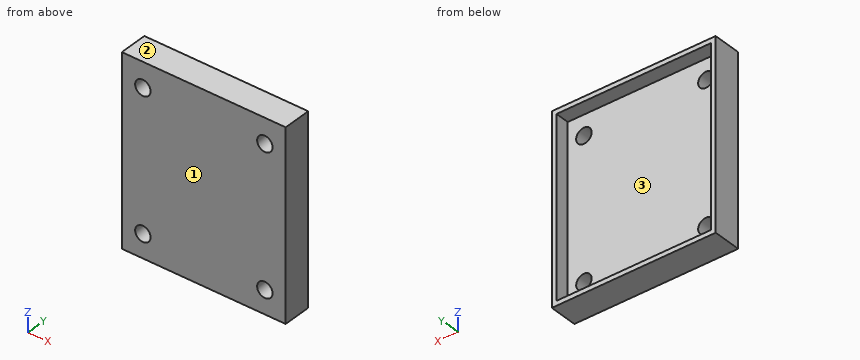
Autodesk Inventor part; units mm, degrees
ref_plane "YZ Plane" through (0, 0, 0) normal (1, 0, 0) x (0, 1, 0)
ref_plane "XZ Plane" through (0, 0, 0) normal (0, 1, 0) x (-1, 0, 0)
ref_plane "XY Plane" through (0, 0, 0) normal (0, 0, 1) x (1, 0, 0)
sketch "Sketch1" plane through (0, 0, 0) normal (0, 1, 0) x (-1, 0, 0)
  line L0 (4.6706, 7.7326) -> (-28.3294, 7.7326)
  line L1 (-28.3294, 7.7326) -> (-28.3294, -32.2674)
  line L2 (-28.3294, -32.2674) -> (4.6706, -32.2674)
  line L3 (4.6706, -32.2674) -> (4.6706, 7.7326)
  point P0 (0, 0)
  dimension "d0" = 33
  dimension "d1" = 40
extrude "Extrusion1" add sketch "Sketch1" along normal blind 3
sketch "Sketch2" plane through (0, 3, 0) normal (0, 1, 0) x (1, 0, 0)
  line L0 (-4.6706, 32.2674) -> (-4.6706, -7.7326)
  line L1 (-4.6706, -7.7326) -> (-4.6706, -4.7326)
  line L2 (-4.6706, -4.7326) -> (-2.8206, -4.7326)
  line L3 (-2.8206, -4.7326) -> (-2.8206, 28.2674)
  line L4 (-2.8206, 28.2674) -> (26.4794, 28.2674)
  line L5 (26.4794, 28.2674) -> (26.4794, -4.7326)
  line L6 (-2.8206, -4.7326) -> (-1.1706, -4.7326)
  line L7 (26.4794, -4.7326) -> (24.8794, -4.7326)
  line L8 (24.8794, -4.7326) -> (24.8794, 28.2674)
  line L9 (-2.8206, 28.2674) -> (-1.1706, 28.2674)
  line L10 (-1.1706, -4.7326) -> (-1.1706, -1.4326)
  line L11 (-1.1706, -1.4326) -> (24.8794, -1.4326)
  point P0 (0, 0)
  dimension "d4" = 3
  dimension "d5" = 1.85
  dimension "d6" = 90
  dimension "d7" = 33
  dimension "d8" = 29.3
  dimension "d9" = 1.65
  dimension "d10" = 1.6
  dimension "d11" = 1.65
  dimension "d26" = 3.3
hole "Hole1" at (-1.1706, 3, 1.4326) at (24.8794, 3, 1.4326) at (24.8794, 3, -28.2674) at (-1.1706, 3, -28.2674) direction (0, -1, 0) diameter 3.3 end through all
sketch "Sketch3" plane through (0, 0, 0) normal (0, -1, 0) x (1, 0, 0)
  line L0 (28.3294, -32.2674) -> (-4.6706, -32.2674)
  line L1 (-4.6706, -32.2674) -> (-5.6706, -32.2674)
  line L2 (-5.6706, -32.2674) -> (-5.6706, -33.2674)
  line L3 (-5.6706, -33.2674) -> (29.3294, -33.2674)
  line L4 (29.3294, -33.2674) -> (29.3294, 8.7326)
  line L5 (28.3294, 7.7326) -> (28.3294, -32.2674)
  line L6 (29.3294, 8.7326) -> (-5.6706, 8.7326)
  line L7 (-5.6706, 8.7326) -> (-5.6706, -32.2674)
  circle A0 centre (24.8794, -28.2674) radius 1.65
  circle A1 centre (-1.1706, -28.2674) radius 1.65
  line L8 (-4.6706, 7.7326) -> (28.3294, 7.7326)
  line L9 (-4.6706, -32.2674) -> (-4.6706, 7.7326)
  line L10 (28.3294, -32.2674) -> (-4.6706, -32.2674)
  line L11 (28.3294, 7.7326) -> (28.3294, -32.2674)
  point P0 (0, 0)
  dimension "d19" = 1
  dimension "d20" = 1
  dimension "d21" = 35
  dimension "d22" = 42
  dimension "d23" = 90
extrude "Extrusion2" add sketch "Sketch3" against normal blind 6 contours L7 L6 L4 L3 L2
sketch "Sketch4" plane through (-5.6706, 0, 8.7326) normal (0, 0, 1) x (1, 0, 0)
  point P0 (5.6706, 0)
sketch "Sketch5" plane through (0, 0, 0) normal (0, -1, 0) x (1, 0, 0)
  line L0 (-5.6706, -33.2674) -> (-5.6706, 8.7326)
  line L1 (-5.6706, 8.7326) -> (-5.6706, 5.7326)
  line L2 (-5.6706, 5.7326) -> (29.3294, 5.7326)
  line L3 (29.3294, -33.2674) -> (29.3294, 8.7326)
  line L4 (29.3294, 8.7326) -> (-5.6706, 8.7326)
  line L5 (-5.6706, 5.7326) -> (-5.6706, 6.7326)
  line L6 (-5.6706, 6.7326) -> (29.3294, 6.7326)
  line L7 (28.3294, 7.7326) -> (-4.6706, 7.7326)
  line L8 (29.3294, 6.7326) -> (29.3294, 5.7326)
  point P0 (0, 0)
  dimension "d27" = 3
  dimension "d28" = 1
extrude "Extrusion3" cut sketch "Sketch5" against normal blind 10 contours L0 L4 L3 L6
extrude "Extrusion4" add sketch "Sketch5" against normal blind 6 contours L0 L6 L3 L2
properties part number "testing holes for circuit board"
Verification items for the finished model (mm, model axes). Face numbers are marked on the shaded views. Coordinates: 2 decimals unless noted, no trailing zeros. Order: outer loops, then holes, each group sorted by start corner. A loop starts at its lowest first (then second) coordinate and runs counter-clockwise, first axis right, second up. Notation, with made-up numbers: (57, -29.5) -> (69, -29.5) arc R38 cw to (69, 8.5) -> close; hole circle Ø11 at (70, 55). An arc over 180 degrees is marked (long way). Use CSV: the item, a comma, the result in double quotes. Start each with the question number.
Q1. Depth check by flat-ended pin: P1, Ø1.5, axis at x = 8.5, z = -9, coming from the +Y side. Enter the tip coordinate at first touch or a pass-through.
Q2. Section check A-A, the plane y = 4.4. Record the cut outline in (x, z), and give its area (3 significant figures).
Q3. Section check C-C, the plane x = 0. Record the cut outline in (y, z), and give its area (3 significant figures).
Q4. Thickness scan on line 1 along X through (y, z) = (3.8, -22); line 2 along Z through (x, y) = (25, 4.45); line 3 along Z through (x, y) = (-2, 0.95). Record the ranges inside material, lowest first.
Q5. Draft check along Z on the marked faces 1, 2 and 3. Enter one of: +Z half, -Z half, draft (parallel to the pull), parting line (faces both ways), or undercut.
Q6. Section check D-D, the plane x = 12. Record the cut outline in (y, z), and give its area (3 significant figures).
Q7. Section check B-B, the plane z = -20. Record the cut outline in (x, y), and give its area (3 significant figures).
Returned:
1,P1,"stops at y = 3"
2,outline,"(-5.67, -33.27) -> (29.33, -33.27) -> (29.33, 6.73) -> (-5.67, 6.73) -> close; hole (-4.67, -32.27) -> (28.33, -32.27) -> (28.33, 5.73) -> (-4.67, 5.73) -> close"
2,area,"146 mm^2"
3,outline,"(0, -33.27) -> (6, -33.27) -> (6, -32.27) -> (3, -32.27) -> (3, -29.43) -> (0, -29.43) -> close; (0, -27.1) -> (3, -27.1) -> (3, 0.27) -> (0, 0.27) -> close; (0, 2.6) -> (3, 2.6) -> (3, 5.73) -> (6, 5.73) -> (6, 6.73) -> (0, 6.73) -> close"
3,area,"112 mm^2"
4,line 1,"x = -5.67 to -4.67, 28.33 to 29.33"
4,line 2,"z = -33.27 to -32.27, 5.73 to 6.73"
4,line 3,"z = -33.27 to -29.69, -26.84 to 0.01, 2.86 to 6.73"
5,face 1,"draft"
5,face 2,"+Z half"
5,face 3,"undercut"
6,outline,"(0, -33.27) -> (6, -33.27) -> (6, -32.27) -> (3, -32.27) -> (3, 5.73) -> (6, 5.73) -> (6, 6.73) -> (0, 6.73) -> close"
6,area,"126 mm^2"
7,outline,"(-5.67, 0) -> (29.33, 0) -> (29.33, 6) -> (28.33, 6) -> (28.33, 3) -> (-4.67, 3) -> (-4.67, 6) -> (-5.67, 6) -> close"
7,area,"111 mm^2"
